from build123d import *

# Parameters (mm, degrees)
SKETCH1_R           = 3.49
SKETCH1_W           = 2.98
SKETCH1_H           = 3.98
BOSS_EXTRUDE2_DEPTH = 7
SKETCH3_R           = 10.198039027
SKETCH3_W           = 11
SKETCH3_H           = 11
BOSS_EXTRUDE3_DEPTH = 50


with BuildPart() as part:
    # Sketch1 → Boss-Extrude2 (new body)
    with BuildSketch(Plane(origin=(0, 0, 0), x_dir=(1, 0, 0), z_dir=(0, 1, 0))):
        with Locations(Location((0, 0, 0), (0, 0, 270))):
            Circle(SKETCH1_R)
        Rectangle(SKETCH1_W, SKETCH1_H, mode=Mode.SUBTRACT)
    extrude(amount=BOSS_EXTRUDE2_DEPTH)

    # Sketch2 → Revolve1 (revolve)
    with BuildSketch(Plane(origin=(0, 0, 0), x_dir=(0, 0, -1), z_dir=(1, 0, 0))):
        with BuildLine():
            Line((10, 3), (12, 3))
            ThreePointArc((12, 3), (11.277776118, 5.080528106), (10.198039027, 7))
            Line((10.198039027, 7), (3.49, 7))
            Line((3.49, 7), (3.49, 6))
            Line((3.49, 6), (8.544003745, 6))
            ThreePointArc((8.544003745, 6), (9.392551236, 4.558506474), (10, 3))
        make_face()
    revolve(axis=Axis((0, 0.002779656, 0), (0, 1, 0)))

    # Sketch3 → Boss-Extrude3 (add)
    with BuildSketch(Plane(origin=(0, 7, 0), x_dir=(1, 0, 0), z_dir=(0, 1, 0))):
        with Locations(Location((0, 0, 0), (0, 0, 90))):
            Circle(SKETCH3_R)
        Rectangle(SKETCH3_W, SKETCH3_H, mode=Mode.SUBTRACT)
    extrude(amount=BOSS_EXTRUDE3_DEPTH)


solid = part.part
Here's how the part is built. I have some questions about the finished solid (model axes, mm). A direction names the side the tool comes from. Coordinates: 2 decimals unless noted, no trailing zeros. Order: outer loops, then holes, each group sorted by start corner. A loop starts at its lowest first (then second) coordinate and runs counter-clockwise, first axis right, second up.
Item 1: If we section it at B-B on z = 0: List the corners of the cut face in (x, y) for me, plus the area to 3 significant figures.
Result sheet:
outline: (-12, 3) - (-10, 3) arc R10.44 cw to (-8.54, 6) - (-3.49, 6) - (-3.49, 0) - (-1.49, 0) - (-1.49, 7) - (-5.5, 7) - (-5.5, 57) - (-10.2, 57) - (-10.2, 7) arc R12.37 ccw to start; (1.49, 0) - (3.49, 0) - (3.49, 6) - (8.54, 6) arc R10.44 cw to (10, 3) - (12, 3) arc R12.37 ccw to (10.2, 7) - (10.2, 57) - (5.5, 57) - (5.5, 7) - (1.49, 7) - close
area: 525 mm2
Item 2: I need wall thicknesses on line 1 (Z direction, x = -0.25, y = 8); line 2 (Y direction, x = -4.5, z = 1); line 3 (X direction, y = 32.5, z = -4). Which ranges of each line are inside material? Lowest first, please.
Result sheet:
line 1: z = -10.19 to -5.5, 5.5 to 10.19
line 2: y = 6 to 7
line 3: x = -9.38 to -5.5, 5.5 to 9.38
Item 3: For P1, Ø2, axis at y = 5, z = 1, coming from the -X side; P2, Ø12, axis at x = 5, y = 29, coming from the -Z side; P3, Ø3, axis at x = 0, z = 6.5, coming from the -Y side, each with a flat end and sliding along its axis, tell me the tip position at first contact or that it passes through.
Result sheet:
P1: stops at x = -11.67
P2: stops at z = -10.2
P3: stops at y = 6
Item 4: If we section it at A-A on x = 0: List the corners of the cut face in (y, z) for me.
Result sheet:
outline: (0, -3.49) - (6, -3.49) - (6, -8.54) arc R10.44 cw to (3, -10) - (3, -12) arc R12.37 ccw to (7, -10.2) - (57, -10.2) - (57, -5.5) - (7, -5.5) - (7, -1.99) - (0, -1.99) - close; (0, 1.99) - (7, 1.99) - (7, 5.5) - (57, 5.5) - (57, 10.2) - (7, 10.2) arc R12.37 ccw to (3, 12) - (3, 10) arc R10.44 cw to (6, 8.54) - (6, 3.49) - (0, 3.49) - close
Item 5: For faces 1 (the face through (0, 57, -7)), 2 (the face through (0, 3, 1.99)), 3 (the face through (3.46, 2.96, -0.45)), 4 (the face through (0, 32, 5.5)), which set-ups out of +Z, -Z, +X, -X, +Y, -Y let a thin tool reach every point of the face, with its end or its side?
Result sheet:
face 1: +Z, -Z, +X, -X, +Y
face 2: +Y, -Y
face 3: -Y
face 4: +Y
Item 6: If we mould it in two halves opening along Z, with no side actions, what happens to faces 5 (the face through (-2, 0, 0)), 6 (the face through (-8.6, 31.65, -5.48)), 7 (the face through (1.49, 3, 0))? For each: +Z half, -Z half, draft (parallel to the pull), parting line (faces both ways), or undercut.
Result sheet:
face 5: draft
face 6: parting line
face 7: undercut
Item 7: If we section it at C-C on y = 28: List the corners of the cut face in (x, z) for me, plus the area to 3 significant figures.
Result sheet:
outline: circle Ø20.4 at (0, 0); hole (-5.5, -5.5) - (5.5, -5.5) - (5.5, 5.5) - (-5.5, 5.5) - close
area: 206 mm2
Item 8: If we section it at D-D on z = 2.75: List the corners of the cut face in (x, y) for me, plus the area to 3 significant figures.
Result sheet:
outline: (-11.68, 3) - (-9.61, 3) arc R10.07 cw to (-8.09, 6) - (-2.15, 6) - (-2.15, 0) - (2.15, 0) - (2.15, 6) - (8.09, 6) arc R10.07 cw to (9.61, 3) - (11.68, 3) arc R12.06 ccw to (9.82, 7) - (9.82, 57) - (5.5, 57) - (5.5, 7) - (-5.5, 7) - (-5.5, 57) - (-9.82, 57) - (-9.82, 7) arc R12.06 ccw to start
area: 491 mm2
